```python
from build123d import *

# Parameters (mm, degrees)
F1_DEPTH = 31.75
F0_W     = 31.75
F0_H     = 31.75
F2_DEPTH = 92.075
F0_H_2   = 88.9
F3_DEPTH = 73.025
F0_R     = 15.875
F4_DEPTH = 53.975


with BuildPart() as f1:
    # F0 (on Top) → F1 (new body)
    with BuildSketch(Plane.XY):
        Polygon((-127, -76.2), (-76.2, -76.2), (-76.2, -44.45), (-76.2, 44.45), (-76.2, 76.2), (-127, 76.2), (-127, 25.4), (-85.725, 25.4), (-85.725, -25.4), (-127, -25.4), align=None)
        Polygon((76.2, -76.2), (127, -76.2), (127, -25.4), (85.725, -25.4), (85.725, 25.4), (127, 25.4), (127, 76.2), (76.2, 76.2), (76.2, 44.45), (76.2, -44.45), align=None)
    extrude(amount=F1_DEPTH)

    # F0 (on Top) → F2 (join)
    with BuildSketch(Plane.XY):
        with Locations((-60.325, 60.325)):
            Rectangle(F0_W, F0_H)
        with Locations((-60.325, -60.325)):
            Rectangle(F0_W, F0_H)
        with Locations((60.325, -60.325)):
            Rectangle(F0_W, F0_H)
        with Locations((60.325, 60.325)):
            Rectangle(F0_W, F0_H)
    extrude(amount=F2_DEPTH)

    # F0 (on Top) → F3 (join)
    with BuildSketch(Plane.XY):
        with Locations((-60.325, 0)):
            Rectangle(F0_W, F0_H_2)
        with Locations((60.325, 0)):
            Rectangle(F0_W, F0_H_2)
    extrude(amount=F3_DEPTH)

    # F0 (on Top) → F4 (join)
    with BuildSketch(Plane.XY):
        Polygon((-44.45, -76.2), (44.45, -76.2), (44.45, -44.45), (44.45, 44.45), (44.45, 76.2), (-44.45, 76.2), (-44.45, 44.45), (-44.45, -44.45), align=None)
        Circle(F0_R, mode=Mode.SUBTRACT)
    extrude(amount=F4_DEPTH)


solid = f1.part
```
Work out the finished part from the listing and answer in its coordinate system (mm). A direction names the side the tool comes from. Round coordinates to 2 decimals unless told otherwise and drop trailing zeros. Write each loop counter-clockwise with the first axis right and the second up, starting at its lowest first coordinate (ties: lowest second). Pieces come first, ordered by that corner, then holes.
1) A cutting plane is placed at C-C on z = 82. Determine the outline of the cut face in (x, y).
2) Determine the mould class of faces 5 (the face through (76.2, -1, 55)), 6 (the face through (44.45, -1, 69)), 7 (the face through (60, 61, 92.075)) for opening direction X: pulls with the +X half, pulls with the -X half, needs draft (parallel to the pull), parting line crosses it, or undercut.
3) Which of the six approach directions +Z, -Z, +X, -X, +Y, -Y give full straight-line access (tool end or side, diameter ignored) to faces 1 (the face through (85.725, 0, 16)), 2 (the face through (-106, -25.4, 16)), 3 (the face through (84, 1, 31.75)), 4 (the face through (-61, 44.45, 82))?
4) A cutting plane is placed at D-D on y = 41. Determine the outline of the cut face in (x, z) (3 decimals), and give its area (3 significant figures).
5) Consider probe 1 along X at (y, z) = (-34, 65); probe 2 along Y at (x, z) = (0, 16) (3 decimals). Determine where each line is inside the solid, lowest interval first.
6) A cutting plane is placed at B-B on x = 0. Determine the outline of the cut face in (y, z) (3 decimals).
7) A cutting plane is placed at A-A on z = 63.5. Determine the outline of the cut face in (x, y), and give its area (3 significant figures).
8) Flat-ended cylindrical pins translate along their axes: P1, Ø6, axis at x = 71, y = 40.5, coming from the +Z side (3 decimals); P2, Ø5, axis at y = 15.5, z = 61.5, coming from the +X side; P3, Ø3, axis at x = 16.5, y = -49.5, coming from the +Z side (3 decimals); P4, Ø5, axis at x = -31, z = 58.5, coming from the +Y side. Find the tip coordinate at first contact, or state that the pin passes through.
Entries:
1. outline: (-76.2, -76.2) - (-44.45, -76.2) - (-44.45, -44.45) - (-76.2, -44.45) - close; (-76.2, 44.45) - (-44.45, 44.45) - (-44.45, 76.2) - (-76.2, 76.2) - close; (44.45, -76.2) - (76.2, -76.2) - (76.2, -44.45) - (44.45, -44.45) - close; (44.45, 44.45) - (76.2, 44.45) - (76.2, 76.2) - (44.45, 76.2) - close
2. face 5: pulls with the +X half
2. face 6: undercut
2. face 7: needs draft
3. face 1: +Z, -Z, +X
3. face 2: +Z, -Z, -X
3. face 3: +Z, +X, +Y, -Y
3. face 4: +Z, +X, -X
4. outline: (-127, 0) - (127, 0) - (127, 31.75) - (76.2, 31.75) - (76.2, 73.025) - (44.45, 73.025) - (44.45, 53.975) - (-44.45, 53.975) - (-44.45, 73.025) - (-76.2, 73.025) - (-76.2, 31.75) - (-127, 31.75) - close
4. area: 12,700 mm2
5. probe 1: x = -76.2 to -44.45, 44.45 to 76.2
5. probe 2: y = -76.2 to -15.875, 15.875 to 76.2
6. outline: (-76.2, 0) - (-15.875, 0) - (-15.875, 53.975) - (-76.2, 53.975) - close; (15.875, 0) - (76.2, 0) - (76.2, 53.975) - (15.875, 53.975) - close
7. outline: (-76.2, -76.2) - (-44.45, -76.2) - (-44.45, 76.2) - (-76.2, 76.2) - close; (44.45, -76.2) - (76.2, -76.2) - (76.2, 76.2) - (44.45, 76.2) - close
7. area: 9,680 mm2
8. P1: stops at z = 73.025
8. P2: stops at x = 76.2
8. P3: stops at z = 53.975
8. P4: passes through
